Can you work these out from the model? Positions are in its coordinate system, mm. A direction names the side the tool comes from. Round coordinates to 2 decimals unless told otherwise and drop trailing zeros. Loops run counter-clockwise (first coordinate to the right, second up) from the corner with the lowest first, then second, coordinate; pieces in that order, holes last. Notation, with made-up numbers: (14.25, -34.75) -> (73.25, -34.75) arc R20 ccw to (73.25, -10.75) -> close; hole circle Ø3 at (10.25, -8.75). An arc over 180 degrees is marked (long way). Answer as a JSON object with one key per item and string values.
```python
from build123d import *

# Parameters (mm, degrees)
F0_R     = 38.1
F0_R_2   = 1.5875
F1_DEPTH = 3.175
F2_DEPTH = 3.175


# Not quite as in the source:
# - a feature names something its author has since deleted; it is built from what else it names


with BuildPart() as f1:
    # F0 (on Front) → F1 (new body)
    with BuildSketch(Plane.XZ):
        Circle(F0_R)
        with BuildLine():
            ThreePointArc((30.5065021635, 12.6362069367), (32.3855299589, 6.441882433), (33.02, 0))
            ThreePointArc((33.02, 0), (32.3855299589, -6.441882433), (30.5065021635, -12.6362069367))
            ThreePointArc((30.5065021635, -12.6362069367), (27.4551265982, -18.3449290943), (23.3486659148, -23.3486659148))
            ThreePointArc((23.3486659148, -23.3486659148), (18.3449290943, -27.4551265982), (12.6362069367, -30.5065021635))
            ThreePointArc((12.6362069367, -30.5065021635), (6.441882433, -32.3855299589), (0, -33.02))
            ThreePointArc((0, -33.02), (-6.441882433, -32.3855299589), (-12.6362069367, -30.5065021635))
            ThreePointArc((-12.6362069367, -30.5065021635), (-18.3449290943, -27.4551265982), (-23.3486659148, -23.3486659148))
            ThreePointArc((-23.3486659148, -23.3486659148), (-27.4551265982, -18.3449290943), (-30.5065021635, -12.6362069367))
            ThreePointArc((-30.5065021635, -12.6362069367), (-32.3855299589, -6.441882433), (-33.02, 0))
            ThreePointArc((-33.02, 0), (-32.3855299589, 6.441882433), (-30.5065021635, 12.6362069367))
            ThreePointArc((-30.5065021635, 12.6362069367), (-27.4551265982, 18.3449290943), (-23.3486659148, 23.3486659148))
            ThreePointArc((-23.3486659148, 23.3486659148), (-18.3449290943, 27.4551265982), (-12.6362069367, 30.5065021635))
            ThreePointArc((-12.6362069367, 30.5065021635), (-6.441882433, 32.3855299589), (0, 33.02))
            ThreePointArc((0, 33.02), (6.441882433, 32.3855299589), (12.6362069367, 30.5065021635))
            ThreePointArc((12.6362069367, 30.5065021635), (18.3449290943, 27.4551265982), (23.3486659148, 23.3486659148))
            ThreePointArc((23.3486659148, 23.3486659148), (27.4551265982, 18.3449290943), (30.5065021635, 12.6362069367))
        make_face(mode=Mode.SUBTRACT)
        with BuildLine():
            ThreePointArc((6.159966783, -2.5515417853), (6.5393858571, -1.300764722), (6.6675, 0))
            ThreePointArc((6.6675, 0), (6.5393858571, 1.300764722), (6.159966783, 2.5515417853))
            ThreePointArc((6.159966783, 2.5515417853), (5.54382364, 3.7042645287), (4.7146344636, 4.7146344636))
            ThreePointArc((4.7146344636, 4.7146344636), (3.7042645287, 5.54382364), (2.5515417853, 6.159966783))
            ThreePointArc((2.5515417853, 6.159966783), (1.300764722, 6.5393858571), (0, 6.6675))
            ThreePointArc((0, 6.6675), (-1.300764722, 6.5393858571), (-2.5515417853, 6.159966783))
            ThreePointArc((-2.5515417853, 6.159966783), (-3.7042645287, 5.54382364), (-4.7146344636, 4.7146344636))
            ThreePointArc((-4.7146344636, 4.7146344636), (-5.54382364, 3.7042645287), (-6.159966783, 2.5515417853))
            ThreePointArc((-6.159966783, 2.5515417853), (-6.5393858571, 1.300764722), (-6.6675, 0))
            ThreePointArc((-6.6675, 0), (-6.5393858571, -1.300764722), (-6.159966783, -2.5515417853))
            ThreePointArc((-6.159966783, -2.5515417853), (-5.54382364, -3.7042645287), (-4.7146344636, -4.7146344636))
            ThreePointArc((-4.7146344636, -4.7146344636), (-3.7042645287, -5.54382364), (-2.5515417853, -6.159966783))
            ThreePointArc((-2.5515417853, -6.159966783), (-1.300764722, -6.5393858571), (0, -6.6675))
            ThreePointArc((0, -6.6675), (1.300764722, -6.5393858571), (2.5515417853, -6.159966783))
            ThreePointArc((2.5515417853, -6.159966783), (3.7042645287, -5.54382364), (4.7146344636, -4.7146344636))
            ThreePointArc((4.7146344636, -4.7146344636), (5.54382364, -3.7042645287), (6.159966783, -2.5515417853))
        make_face()
        Circle(F0_R_2, mode=Mode.SUBTRACT)
        with BuildLine():
            ThreePointArc((0, -33.02), (6.441882433, -32.3855299589), (12.6362069367, -30.5065021635))
            Line((12.6362069367, -30.5065021635), (2.5515417853, -6.159966783))
            ThreePointArc((2.5515417853, -6.159966783), (1.300764722, -6.5393858571), (0, -6.6675))
            Line((0, -6.6675), (0, -33.02))
        make_face()
    extrude(amount=F1_DEPTH)

    # F0 (on Front) → F2 (join)
    with BuildSketch(Plane.XZ):
        Circle(F0_R)
        with BuildLine():
            ThreePointArc((30.5065021635, 12.6362069367), (32.3855299589, 6.441882433), (33.02, 0))
            ThreePointArc((33.02, 0), (32.3855299589, -6.441882433), (30.5065021635, -12.6362069367))
            ThreePointArc((30.5065021635, -12.6362069367), (27.4551265982, -18.3449290943), (23.3486659148, -23.3486659148))
            ThreePointArc((23.3486659148, -23.3486659148), (18.3449290943, -27.4551265982), (12.6362069367, -30.5065021635))
            ThreePointArc((12.6362069367, -30.5065021635), (6.441882433, -32.3855299589), (0, -33.02))
            ThreePointArc((0, -33.02), (-6.441882433, -32.3855299589), (-12.6362069367, -30.5065021635))
            ThreePointArc((-12.6362069367, -30.5065021635), (-18.3449290943, -27.4551265982), (-23.3486659148, -23.3486659148))
            ThreePointArc((-23.3486659148, -23.3486659148), (-27.4551265982, -18.3449290943), (-30.5065021635, -12.6362069367))
            ThreePointArc((-30.5065021635, -12.6362069367), (-32.3855299589, -6.441882433), (-33.02, 0))
            ThreePointArc((-33.02, 0), (-32.3855299589, 6.441882433), (-30.5065021635, 12.6362069367))
            ThreePointArc((-30.5065021635, 12.6362069367), (-27.4551265982, 18.3449290943), (-23.3486659148, 23.3486659148))
            ThreePointArc((-23.3486659148, 23.3486659148), (-18.3449290943, 27.4551265982), (-12.6362069367, 30.5065021635))
            ThreePointArc((-12.6362069367, 30.5065021635), (-6.441882433, 32.3855299589), (0, 33.02))
            ThreePointArc((0, 33.02), (6.441882433, 32.3855299589), (12.6362069367, 30.5065021635))
            ThreePointArc((12.6362069367, 30.5065021635), (18.3449290943, 27.4551265982), (23.3486659148, 23.3486659148))
            ThreePointArc((23.3486659148, 23.3486659148), (27.4551265982, 18.3449290943), (30.5065021635, 12.6362069367))
        make_face(mode=Mode.SUBTRACT)
        with BuildLine():
            ThreePointArc((-23.3486659148, -23.3486659148), (-18.3449290943, -27.4551265982), (-12.6362069367, -30.5065021635))
            Line((-12.6362069367, -30.5065021635), (-2.5515417853, -6.159966783))
            ThreePointArc((-2.5515417853, -6.159966783), (-3.7042645287, -5.54382364), (-4.7146344636, -4.7146344636))
            Line((-4.7146344636, -4.7146344636), (-23.3486659148, -23.3486659148))
        make_face()
        with BuildLine():
            ThreePointArc((-33.02, 0), (-32.3855299589, -6.441882433), (-30.5065021635, -12.6362069367))
            Line((-30.5065021635, -12.6362069367), (-6.159966783, -2.5515417853))
            ThreePointArc((-6.159966783, -2.5515417853), (-6.5393858571, -1.300764722), (-6.6675, 0))
            Line((-6.6675, 0), (-33.02, 0))
        make_face()
        with BuildLine():
            Line((-4.7146344636, 4.7146344636), (-23.3486659148, 23.3486659148))
            ThreePointArc((-23.3486659148, 23.3486659148), (-27.4551265982, 18.3449290943), (-30.5065021635, 12.6362069367))
            Line((-30.5065021635, 12.6362069367), (-6.159966783, 2.5515417853))
            ThreePointArc((-6.159966783, 2.5515417853), (-5.54382364, 3.7042645287), (-4.7146344636, 4.7146344636))
        make_face()
        with BuildLine():
            Line((0, 6.6675), (0, 33.02))
            ThreePointArc((0, 33.02), (-6.441882433, 32.3855299589), (-12.6362069367, 30.5065021635))
            Line((-12.6362069367, 30.5065021635), (-2.5515417853, 6.159966783))
            ThreePointArc((-2.5515417853, 6.159966783), (-1.300764722, 6.5393858571), (0, 6.6675))
        make_face()
        with BuildLine():
            Line((4.7146344636, 4.7146344636), (23.3486659148, 23.3486659148))
            ThreePointArc((23.3486659148, 23.3486659148), (18.3449290943, 27.4551265982), (12.6362069367, 30.5065021635))
            Line((12.6362069367, 30.5065021635), (2.5515417853, 6.159966783))
            ThreePointArc((2.5515417853, 6.159966783), (3.7042645287, 5.54382364), (4.7146344636, 4.7146344636))
        make_face()
        with BuildLine():
            Line((6.6675, 0), (33.02, 0))
            ThreePointArc((33.02, 0), (32.3855299589, 6.441882433), (30.5065021635, 12.6362069367))
            Line((30.5065021635, 12.6362069367), (6.159966783, 2.5515417853))
            ThreePointArc((6.159966783, 2.5515417853), (6.5393858571, 1.300764722), (6.6675, 0))
        make_face()
        with BuildLine():
            ThreePointArc((23.3486659148, -23.3486659148), (27.4551265982, -18.3449290943), (30.5065021635, -12.6362069367))
            Line((30.5065021635, -12.6362069367), (6.159966783, -2.5515417853))
            ThreePointArc((6.159966783, -2.5515417853), (5.54382364, -3.7042645287), (4.7146344636, -4.7146344636))
            Line((4.7146344636, -4.7146344636), (23.3486659148, -23.3486659148))
        make_face()
    extrude(amount=F2_DEPTH)


solid = f1.part
```
Q1. I want a section at B-B, the plane x = -21. Write out the boundary of the cut face in (y, z) (3 decimals), then the cut area to 3 significant figures.
Determined:
{"outline": "(-3.175, -31.79) -> (0, -31.79) -> (0, -21) -> (-3.175, -21) -> close; (-3.175, -8.698) -> (0, -8.698) -> (0, 0) -> (-3.175, 0) -> close; (-3.175, 8.698) -> (0, 8.698) -> (0, 21) -> (-3.175, 21) -> close; (-3.175, 25.482) -> (0, 25.482) -> (0, 31.79) -> (-3.175, 31.79) -> close", "area": "121 mm²"}
Q2. I want a section at C-C, the plane z = -17.5. Write out the boundary of the cut face in (x, y) (3 decimals).
Determined:
{"outline": "(-33.843, -3.175) -> (-28.001, -3.175) -> (-28.001, 0) -> (-33.843, 0) -> close; (-17.5, -3.175) -> (-7.249, -3.175) -> (-7.249, 0) -> (-17.5, 0) -> close; (0, -3.175) -> (7.249, -3.175) -> (7.249, 0) -> (0, 0) -> close; (17.5, -3.175) -> (33.843, -3.175) -> (33.843, 0) -> (17.5, 0) -> close"}
Q3. I'm going to push flat-ended pins straight in: pin 1 (1.6 mm diameter, centred on y = -2, z = 22.5, fed in from +X); pin 2 (1.6 mm diameter, centred on y = -2, z = -15.5, fed in from -X); pin 3 (1 mm diameter, centred on x = -26, y = -1.5, fed in from +Z). Where does each tip first touch, or does it pass through?
Determined:
{"pin 1": "x = 31.32", "pin 2": "x = -35.15", "pin 3": "z = 28.31"}
Q4. If I drill on L1, parallel to X at y = -2, z = -26; L2, parallel to X at y = -2.85, z = -20; L3, parallel to X at y = -0.15, z = 8.5, over which ranges is the centre line in solid material (lowest first)? Write a range as [from, to].
Determined:
{"L1": "[-27.85, -10.77], [0, 10.77], [20.35, 27.85]", "L2": "[-32.43, -26.27], [-20, -8.28], [0, 8.28], [20, 32.43]", "L3": "[-37.14, -31.91], [-20.52, -8.5], [-3.52, 0], [3.52, 8.5], [20.52, 37.14]"}
Q5. We'd pull the mould along X, two halves only. Please class faces 1 (the cylindrical face through (6.536, -1.565, -1.319)), 2 (the cylindrical face through (-30.235, -1.565, -23.183)), 3 (the flat face through (8, 0, 1)): pulls with the +X half, pulls with the -X half, needs draft (parallel to the pull), parting line crosses it, or undercut.
Determined:
{"face 1": "undercut", "face 2": "parting line crosses it", "face 3": "needs draft"}
Q6. I want a section at A-A, the plane y = -0.85. Give the number of separate pieces and of enclosed holes in the cut face, then the cut area to 3 significant figures.
Determined:
{"separate pieces": "1", "enclosed holes": "9", "area": "2,910 mm²"}
Q7. On a 3-axis mill with a long thin cutter (end or side, diameter ignored), from which of +Z, -Z, +X, -X, +Y, -Y can I reach the whole of each face in a straight line? I mean faces 4 (the flat face through (7.664, -1.565, -18.504)), 5 (the flat face through (8, -3.175, 1)). Say none if no direction works.
Determined:
{"face 4": "+Y, -Y", "face 5": "+Z, -Z, +X, -X, -Y"}
